Could you check a few things on this model? Use its own coordinates, in mm. A direction names the side the tool comes from. Round coordinates to 2 decimals unless told otherwise and drop trailing zeros. Loops run counter-clockwise (first coordinate to the right, second up) from the corner with the lowest first, then second, coordinate; pieces in that order, holes last. Notation, with made-up numbers: (46, 69.5) - (61, 69.5) arc R26 ccw to (61, 107.5) - close; hole circle Ø4 at (-24, -26). An arc over 180 degrees is marked (long way). Use one line per item in the form item = value.
```python
from build123d import *

# Parameters (mm, degrees)
SKETCH_1_R          = 15
EXTRUDE_1_DEPTH     = 3
SKETCH_2_R          = 10
EXTRUDE_2_DEPTH     = 12
SKETCH_3_R          = 1.3
CUT_EXTRUDE_1_DEPTH = 6
SKETCH_4_R          = 2
CUT_EXTRUDE_2_DEPTH = 6
CHAMFER_1_SIZE      = 0.5


with BuildPart() as part:
    # 草图1 → 凸台-拉伸1 (new body)
    with BuildSketch(Plane.XY):
        Circle(SKETCH_1_R)
    extrude(amount=EXTRUDE_1_DEPTH)

    # 草图2 → 凸台-拉伸2 (add)
    with BuildSketch(Plane.XY.offset(3)):
        Circle(SKETCH_2_R)
    extrude(amount=EXTRUDE_2_DEPTH)

    # 草图3 → 切除-拉伸1 (cut)
    with BuildSketch(Plane.XY.offset(15)):
        with Locations((-6.999, -0.001)):
            Circle(SKETCH_3_R)
        with Locations((0, 7)):
            Circle(SKETCH_3_R)
        with Locations((0.002, -7)):
            Circle(SKETCH_3_R)
        with Locations((7.001, 0.001)):
            Circle(SKETCH_3_R)
    extrude(amount=-CUT_EXTRUDE_1_DEPTH, mode=Mode.SUBTRACT)

    # 草图4 → 切除-拉伸2 (cut)
    with BuildSketch(Plane(origin=(0, 0, 0), x_dir=(-1, 0, 0), z_dir=(0, 0, -1))):
        with Locations((0, -5)):
            Circle(SKETCH_4_R)
        with Locations((-4.328627019, 2.500866025)):
            Circle(SKETCH_4_R)
        with Locations((4.331627019, 2.499133975)):
            Circle(SKETCH_4_R)
    extrude(amount=-CUT_EXTRUDE_2_DEPTH, mode=Mode.SUBTRACT)

    # 倒角1
    chamfer_1_edges = [part.edges().sort_by_distance(p)[0] for p in [
        (-15, 0, 0),
        (-15, 0, 3),
        (-10, 0, 15),
    ]]
    chamfer(chamfer_1_edges, length=CHAMFER_1_SIZE)


solid = part.part
```
1. We'd pull the mould along Y, two halves only. Please class faces 4 (the face through (0, 0, 0)), 5 (the face through (-14.985, 0.66, 1.486)), 6 (the face through (0, -5, 6)): +Y half, -Y half, draft (parallel to the pull), parting line (faces both ways), or undercut.
Solution:
face_4 = draft
face_5 = parting line
face_6 = undercut
2. If we section it at B-B, the plane z = 10.25: Write out the boundary of the cut face in (x, y), plus the area to 3 significant figures.
Solution:
outline = circle Ø20 at (0, 0); hole circle Ø2.6 at (-7, 0); hole circle Ø2.6 at (0, -7); hole circle Ø2.6 at (0, 7); hole circle Ø2.6 at (7, 0)
area = 293 mm^2
3. On a 3-axis mill with a long thin cutter (end or side, diameter ignored), from which of +Z, -Z, +X, -X, +Y, -Y can I reach the whole of each face in a straight line? I mean faces 1 (the face through (5.702, 0.058, 12.042)), 2 (the face through (0, -7, 3)), 3 (the face through (0, 0, 15)). Say none if no direction works.
Solution:
face_1 = +Z
face_2 = -Z
face_3 = +Z, +X, -X, +Y, -Y
4. For P1, Ø1.2, axis at x = -5, y = 3, coming from the -Z side; P2, Ø0.8, axis at x = -0.5, y = -6.5, coming from the +Z side; P3, Ø4, axis at y = 4, z = 12, coming from the +X side, each with a flat end and sliding along its axis, tell me the tip position at first contact or that it passes through.
Solution:
P1 = 6
P2 = 9
P3 = 9.8
5. Please list where these lines run through material, in increasing order: line 1 along Z through (x, y) = (12.25, 3.75); line 2 along Y through (x, z) = (4.25, 1.25); line 3 along X through (y, z) = (-6.25, 9.75).
Solution:
line_1 = 0 to 3
line_2 = -14.39 to 0.5, 4.5 to 14.39
line_3 = -7.81 to -1.06, 1.06 to 7.81
6. If we section it at C-C, the plane z = 1: Write out the boundary of the cut face in (x, y).
Solution:
outline = circle Ø30 at (0, 0); hole circle Ø4 at (-4.33, 2.5); hole circle Ø4 at (0, -5); hole circle Ø4 at (4.33, 2.5)
7. If we section it at A-A, the plane x = 0: Write out the boundary of the cut face in (y, z).
Solution:
outline = (-15, 0.5) - (-14.5, 0) - (-7, 0) - (-7, 6) - (-3, 6) - (-3, 0) - (14.5, 0) - (15, 0.5) - (15, 2.5) - (14.5, 3) - (10, 3) - (10, 14.5) - (9.5, 15) - (8.3, 15) - (8.3, 9) - (5.7, 9) - (5.7, 15) - (-5.7, 15) - (-5.7, 9) - (-8.3, 9) - (-8.3, 15) - (-9.5, 15) - (-10, 14.5) - (-10, 3) - (-14.5, 3) - (-15, 2.5) - close
